Autodesk Inventor part; units mm, degrees
ref_plane "YZ Plane" through (0, 0, 0) normal (1, 0, 0) x (0, 1, 0)
ref_plane "XZ Plane" through (0, 0, 0) normal (0, 1, 0) x (-1, 0, 0)
ref_plane "XY Plane" through (0, 0, 0) normal (0, 0, 1) x (1, 0, 0)
sketch "Sketch1" plane through (0, 0, 0) normal (0, 1, 0) x (-1, 0, 0)
  line L0 (14.5266, 28.8729) -> (-12.4734, 28.8729)
  line L1 (-12.4734, 28.8729) -> (-12.4734, -42.1271)
  line L2 (-12.4734, -42.1271) -> (14.5266, -42.1271)
  line L3 (14.5266, -42.1271) -> (14.5266, 28.8729)
  point P0 (0, 0)
  dimension "d0" = 71
  dimension "d1" = 27
extrude "Extrusion1" add sketch "Sketch1" along normal blind 3
sketch "Sketch2" plane through (0, 3, 0) normal (0, 1, 0) x (1, 0, 0)
  circle A0 centre (-11.5266, -15.8729) radius 1.5
  line L0 (-14.5266, -28.8729) -> (12.4734, -28.8729)
  line L1 (-14.5266, 42.1271) -> (-14.5266, -28.8729)
  circle A1 centre (-11.5266, 39.1271) radius 1.5
  circle A2 centre (9.4734, -15.8729) radius 1.5
  circle A3 centre (9.4734, 39.1271) radius 1.5
  point P0 (0, 0)
  dimension "d4" = 3
  dimension "d5" = 3
  dimension "d6" = 13
  dimension "d9" = 55
  dimension "d12" = 21
extrude "Extrusion2" cut sketch "Sketch2" against normal through all
properties part number "k2_t2_base"
Geometry: final body of the model. Coordinates: model frame, mm. Coordinates: 2 decimals unless noted, no trailing zeros. Order: outer loops, then holes, each group sorted by start corner. A loop starts at its lowest first (then second) coordinate and runs counter-clockwise, first axis right, second up. Notation, with made-up numbers: M 44,54 L 87,54 A16 cw 87,66 Z; hole C 39.5,16.5 d1. An arc over 180 degrees is marked long. Answer in a Markdown table with one row per item. Add a question column.
Q1. Line query: L1, parallel to Z at x = 8.75, y = 0.8; L2, parallel to Z at x = 10.75, y = 1.2. Output: solid intervals per line, ascending.
Q2. Mould query, pull axis Z, two halves, no side actions, for faces 1 (the flat face through (-1, 3, -6)), 2 (the cylindrical face through (-12.717, 1.521, -38.214)), 3 (the flat face through (-1, 1, -42.127)). Classes: released by +Z, released by -Z, zero draft, split by the parting line, or undercut.
Q3. Section query A-A on x = -12. Return the cut outline in (y, z).
Q4. Contact query for flat-ended pins moving along their axis: P1, Ø5, axis at x = -11.53, z = 15.87, coming from the -Y side; P2, Ø2.5, axis at x = -11.53, z = -39.13, coming from the +Y side. Output: stop coordinate, or through.
Completed:
| question | item | result |
|---|---|---|
| 1 | L1 | z = -42.13 to -40.44, -37.81 to 14.56, 17.19 to 28.87 |
| 1 | L2 | z = -42.13 to -39.91, -38.34 to 15.09, 16.66 to 28.87 |
| 2 | face 1 | zero draft |
| 2 | face 2 | undercut |
| 2 | face 3 | released by -Z |
| 3 | outline | M 0,-42.13 L 3,-42.13 L 3,-40.55 L 0,-40.55 Z; M 0,-37.7 L 3,-37.7 L 3,14.45 L 0,14.45 Z; M 0,17.3 L 3,17.3 L 3,28.87 L 0,28.87 Z |
| 4 | P1 | stops at y = 0 |
| 4 | P2 | passes through |
